Design review of the part built by this model. Coordinates are the model's own, in mm. A direction names the side the tool comes from. Give positions to 0.01 mm unless a question says otherwise; leave off trailing zeros. Order: outer loops, then holes, each group sorted by start corner. A loop starts at its lowest first (then second) coordinate and runs counter-clockwise, first axis right, second up. Notation, with made-up numbers: (81.25, 12.5) -> (137.25, 12.5) arc R9 ccw to (137.25, 24.5) -> close; hole circle Ø10 at (18.5, -17). An arc over 180 degrees is marked (long way). Answer in a Markdown table with one row per item. Add a question column.
```python
from build123d import *

# Parameters (mm, degrees)
REVOLUTION_ANGLE = -180
SKETCH001_R      = 1.5
PAD_DEPTH        = 4.5
POCKET_DEPTH     = 2
SKETCH003_R      = 2.8
POCKET001_DEPTH  = 2


with BuildPart() as part:
    # Sketch → Revolution (revolve)
    with BuildSketch(Plane.XZ):
        Polygon((13.4, 4.5), (13.4, 2.5), (13.9, 2), (13.9, 0), (14.7, 0), (14.7, 8), (13.9, 8), (13.9, 5), align=None)
    revolve(axis=Axis((0, 0, 0), (0, 0, 1)), revolution_arc=REVOLUTION_ANGLE)

    # Sketch001 (on Face10 of Revolution) → Pad (new body)
    with BuildSketch(Plane(origin=(0, 0, 0), x_dir=(1, 0, 0), z_dir=(0, 1, 0))):
        with BuildLine():
            ThreePointArc((18.9, -8), (22.9, -4), (18.9, 0))
            Line((18.9, 0), (13.9, 0))
            Line((13.9, 0), (13.9, -8))
            Line((13.9, -8), (18.9, -8))
        make_face()
        with Locations((18.9, -4)):
            Circle(SKETCH001_R, mode=Mode.SUBTRACT)
        with BuildLine():
            ThreePointArc((-18.9, 0), (-22.9, -4), (-18.9, -8))
            Line((-18.9, -8), (-13.9, -8))
            Line((-13.9, -8), (-13.9, 0))
            Line((-13.9, 0), (-18.9, 0))
        make_face()
        with Locations((-18.9, -4)):
            Circle(SKETCH001_R, mode=Mode.SUBTRACT)
    extrude(amount=-PAD_DEPTH)

    # Sketch002 → Pocket (cut)
    with BuildSketch(Plane.XZ.offset(5)):
        Polygon((21.65, 2.412287), (21.65, 5.587713), (18.9, 7.175426), (16.15, 5.587713), (16.15, 2.412287), (18.9, 0.824574), align=None)
    extrude(amount=-POCKET_DEPTH, mode=Mode.SUBTRACT)

    # Sketch003 (on Face28 of Pocket) → Pocket001 (cut)
    with BuildSketch(Plane.XZ.offset(4.5)):
        with Locations((-18.9, 4)):
            Circle(SKETCH003_R)
    extrude(amount=-POCKET001_DEPTH, mode=Mode.SUBTRACT)


solid = part.part
```
1) Machinability: for faces 5 (the face through (-15.5, -4.5, 3.9)), 6 (the face through (-17.7, -2.5, 2.8)), 7 (the face through (0.306, -13.897, 0.986)), which of the approach directions +Z, -Z, +X, -X, +Y, -Y give a long, thin tool a straight path to every point of the face, cutting with its end or side? Answer none if there is none.
2) For L1, parallel to X at y = -1.5, z = 4; L2, parallel to Z at x = -18.9, y = -1.8; L3, parallel to X at y = -1, z = 2.75, list the stretches that pass through material, from the lowest coordinate up.
3) Mouldability with a two-part tool opening along X and no side actions: class faces 1 (the face through (-22.9, -2.2, 3.9)), 2 (the face through (22.9, -2.2, 4.1)), 3 (the face through (21.65, -4, 4)), 4 (the face through (17, 0, 4)) as +X half, -X half, draft (parallel to the pull), parting line (faces both ways), or undercut.
4) Add section B-B, the plane z = 6. Write out the cut boundary in (x, y).
5) Clearance check with flat-ended pins moving along their axes: P1, Ø4, axis at y = -6, z = 2.5, coming from the -X side; P2, Ø2.5, axis at x = 19, z = 2.5, coming from the -Y side; P3, Ø4.5, axis at x = 17.5, z = 2.5, coming from the -Y side. State where each tip first meets the part, or that it passes through.
6) Add section A-A, the plane y = -4. Give the number of separate pieces and of enclosed holes in the cut face, and give its area (3 significant figures).
Verdict:
| question | item | result |
|---|---|---|
| 1 | face 5 | +Z, -Z, -X, -Y |
| 1 | face 6 | -Y |
| 1 | face 7 | -Z, +Y |
| 2 | L1 | x = -22.9 to -20.4, -17.4 to -13.32, 13.32 to 17.4, 20.4 to 22.9 |
| 2 | L2 | z = 0 to 2.5, 5.5 to 8 |
| 2 | L3 | x = -22.7 to -19.73, -18.07 to -13.36, 13.36 to 18.07, 19.73 to 22.7 |
| 3 | face 1 | -X half |
| 3 | face 2 | +X half |
| 3 | face 3 | undercut |
| 3 | face 4 | draft |
| 4 | outline | (-22.36, -4.5) -> (-20.86, -4.5) -> (-20.86, -2.5) -> (-16.94, -2.5) -> (-16.94, -4.5) -> (-13.99, -4.5) arc R14.7 ccw to (13.99, -4.5) -> (16.86, -4.5) -> (16.86, -3) -> (20.94, -3) -> (20.94, -4.5) -> (22.36, -4.5) -> (22.36, 0) -> (13.9, 0) arc R13.9 cw to (-13.9, 0) -> (-22.36, 0) -> close |
| 5 | P1 | stops at x = -22.9 |
| 5 | P2 | stops at y = -3 |
| 5 | P3 | stops at y = -4.5 |
| 6 | separate pieces | 2 |
| 6 | enclosed holes | 2 |
| 6 | area | 91.5 mm2 |
